from build123d import *

# Parameters (mm, degrees)
F0_W          = 2600
F0_H          = 1200
F0_W_2        = 1200
F0_H_2        = 1100
F1_DEPTH      = 100
F2_W          = 40
F2_H          = 80
F3_DEPTH      = 2600.001
F4_W          = 40
F4_H          = 80
F5_DEPTH      = 1160.001
F6_W          = 90
F6_H          = 80
F7_DEPTH      = 550
F7_DEPTH_BACK = 550
F8_W          = 40
F8_H          = 1200
F9_DEPTH      = 60
F10_W         = 35
F10_H         = 55
F11_DEPTH     = 1200.001


with BuildPart() as f1:
    # F0 (on Top) → F1 (new body)
    with BuildSketch(Plane.XY):
        Rectangle(F0_W, F0_H)
        with Locations((-625, 0)):
            Rectangle(F0_W_2, F0_H_2, mode=Mode.SUBTRACT)
        with Locations((625, 0)):
            Rectangle(F0_W_2, F0_H_2, mode=Mode.SUBTRACT)
    extrude(amount=F1_DEPTH)

    # F2 (on face) → F3 (cut, through all)
    with BuildSketch(Plane(origin=(-1300, 0, 0), x_dir=(0, -1, 0), z_dir=(-1, 0, 0))):
        with Locations((-580, 50)):
            Rectangle(F2_W, F2_H)
        with Locations((580, 50)):
            Rectangle(F2_W, F2_H)
    extrude(amount=-F3_DEPTH, mode=Mode.SUBTRACT)

    # F4 (on face) → F5 (cut, through all)
    with BuildSketch(Plane.XZ.offset(560)):
        with Locations((1280, 50)):
            Rectangle(F4_W, F4_H)
        with Locations((-1280, 50)):
            Rectangle(F4_W, F4_H)
    extrude(amount=-F5_DEPTH, mode=Mode.SUBTRACT)

    # F6 (on Front) → F7 (cut, two sides)
    with BuildSketch(Plane.XZ) as f7_sk:
        with Locations((-45, 50)):
            Rectangle(F6_W, F6_H)
    extrude(amount=-F7_DEPTH, mode=Mode.SUBTRACT)
    extrude(f7_sk.sketch, amount=F7_DEPTH_BACK, mode=Mode.SUBTRACT)

    # F8 (on face) → F9 (join)
    with BuildSketch(Plane.XY.offset(100)):
        with Locations((-1280, 0)):
            Rectangle(F8_W, F8_H)
        with Locations((1280, 0)):
            Rectangle(F8_W, F8_H)
    extrude(amount=F9_DEPTH)

    # F10 (on face) → F11 (cut, through all)
    with BuildSketch(Plane.XZ.offset(600)):
        with Locations((1280.4266214371, 130)):
            Rectangle(F10_W, F10_H)
        with Locations((-1280.4266214371, 130)):
            Rectangle(F10_W, F10_H)
    extrude(amount=-F11_DEPTH, mode=Mode.SUBTRACT)


solid = f1.part
Design review of the part built by this model. Coordinates are the model's own, in mm. A direction names the side the tool comes from. Coordinates: 2 decimals unless noted, no trailing zeros. Write each loop counter-clockwise with the first axis right and the second up, starting at its lowest first coordinate (ties: lowest second). Pieces come first, ordered by that corner, then holes. Notation, with made-up numbers: (50, 87) - (60, 87) arc R9 ccw to (60, 94) - close; hole circle Ø3 at (-38.75, 20.25). An arc over 180 degrees is marked (long way). One line per item, written item: value.
1) Mouldability with a two-part tool opening along Z and no side actions: class faces 5 (the face through (-6, 581, 10)), 6 (the face through (-6, 600, 94)), 7 (the face through (-1260, -8, 49)), 8 (the face through (-6, 3, 100)) as +Z half, -Z half, draft (parallel to the pull), parting line (faces both ways), or undercut.
Answer sheet:
face 5: undercut
face 6: draft
face 7: undercut
face 8: +Z half
2) Add section B-B (x = 1074). State the section outline as (y, z) points, plus the area to 3 significant figures.
Answer sheet:
outline: (-600, 0) - (-550, 0) - (-550, 100) - (-600, 100) - (-600, 90) - (-560, 90) - (-560, 10) - (-600, 10) - close; (550, 0) - (600, 0) - (600, 10) - (560, 10) - (560, 90) - (600, 90) - (600, 100) - (550, 100) - close
area: 3,600 mm2
3) For faces 1 (the face through (0, -8, 49)), 2 (the face through (1260, -8, 130)), 3 (the face through (1260, -8, 49)), 4 (the face through (1225, -8, 49)), list the 3-axis set-ups (+Z, -Z, +X, -X, +Y, -Y) from which the entire face can be reached by the end or side of a thin tool; tool diameter is ignored.
Answer sheet:
face 1: none
face 2: +Z, +Y, -Y
face 3: +X, +Y, -Y
face 4: +Z, -Z
4) Add section C-C (y = 162). Give the number of separate pieces and of enclosed holes in the cut face, plus the area to 4 significant figures.
Answer sheet:
separate pieces: 3
enclosed holes: 2
area: 12,550 mm2
5) Add section A-A (z = 132.5). State the section outline as (x, y) points.
Answer sheet:
outline: (-1300, -600) - (-1297.93, -600) - (-1297.93, 600) - (-1300, 600) - close; (-1262.93, -600) - (-1260, -600) - (-1260, 600) - (-1262.93, 600) - close; (1260, -600) - (1262.93, -600) - (1262.93, 600) - (1260, 600) - close; (1297.93, -600) - (1300, -600) - (1300, 600) - (1297.93, 600) - close
6) Insertion check: pin 1 (12 mm diameter, centred on y = 363.5, z = 51, fed in from -X); pin 2 (1.5 mm diameter, centred on y = -471.5, z = 42.5, fed in from +X); pin 3 (8 mm diameter, centred on x = 228, z = 41.5, fed in from -Y). Each pin has a flat end and moves straight along its axis. Give the tip position at first contact, or say it passes through.
Answer sheet:
pin 1: stops at x = -1260
pin 2: stops at x = 1260
pin 3: stops at y = -560
7) To check wall thickness, follow probe 1 along X at (y, z) = (479, 77.5); probe 2 along Y at (x, z) = (-90, 83); probe 3 along Y at (x, z) = (920, 95.5). State the ranges of each line that lie inside material, in increasing order.
Answer sheet:
probe 1: x = -1260 to -1225, 0 to 25, 1225 to 1260
probe 2: y = -560 to -550, 550 to 560
probe 3: y = -600 to -550, 550 to 600
